Input: part model. Units: mm. Frame: model coordinates. A direction names the side the tool comes from. Round coordinates to 2 decimals unless told otherwise and drop trailing zeros. Loops run counter-clockwise (first coordinate to the right, second up) from the corner with the lowest first, then second, coordinate; pieces in that order, holes last. Notation, with made-up numbers: (-10.75, -16.75) -> (24.25, -16.75) arc R13 cw to (24.25, -2.75) -> close; hole circle Ø2 at (10.25, 12). An arc over 180 degrees is marked (long way). Answer in a Markdown table with one row per item. Add a question column.
Q1. Section A-A, the plane x = 0.9. Output: boundary loops of the cut face in (y, z), and give its area (3 significant figures).
Q2. Section D-D, the plane x = -0.65. Output: boundary loops of the cut face in (y, z).
Q3. Pin query (flat end, axial travel): pin 1 (0.8 mm diameter, centred on x = 0.5, y = -2, fed in from -Z); pin 2 (1.5 mm diameter, centred on y = -5, z = -3.5, fed in from -X). Return the tip coordinate at first contact, or that it passes through.
Q4. Section B-B, the plane z = -3.85. Output: boundary loops of the cut face in (x, y).
Q5. Ray query, L1, parallel to X at y = -5.75, z = -3.5; L2, parallel to Y at x = -0.15, z = -4.6; L3, parallel to Z at x = 1.05, y = -5. Return the intervals inside material, ascending. Write a range as from..to.
Q6. Section C-C, the plane y = -4.5. Output: boundary loops of the cut face in (x, z), and give its area (3 significant figures).
Q7. Reachability of faces 1 (the face through (0, -3, -2.346)), 2 (the face through (-0.362, -3, -3)), 3 (the face through (1.138, -3, -3)) from +Z, -Z, +X, -X, +Y, -Y: full face, straight path, thin tool, end or side. Return the list, or none.
```python
from build123d import *

# Parameters (mm, degrees)
F0_W     = 1.5
F0_H     = 2
F1_DEPTH = 6
F2_W     = 2.5
F2_H     = 3
F3_DEPTH = 1
F4_DEPTH = 1


with BuildPart() as f1:
    # F0 (on Front) → F1 (new body)
    with BuildSketch(Plane.XZ):
        with Locations((0.387931, -3.345636)):
            Rectangle(F0_W, F0_H)
    extrude(amount=F1_DEPTH)

    # F2 (on face) → F3 (join)
    with BuildSketch(Plane.XZ.offset(6)):
        with Locations((0.387931, -3.345636)):
            Rectangle(F2_W, F2_H)
    extrude(amount=F3_DEPTH)

    # F2 (on face) → F4 (join)
    with BuildSketch(Plane.XZ.offset(6)):
        with Locations((0.387931, -3.345636)):
            Rectangle(F2_W, F2_H)
    extrude(amount=F4_DEPTH)


solid = f1.part
```
Answer block:
| question | item | result |
|---|---|---|
| 1 | outline | (-7, -4.85) -> (-6, -4.85) -> (-6, -4.35) -> (0, -4.35) -> (0, -2.35) -> (-6, -2.35) -> (-6, -1.85) -> (-7, -1.85) -> close |
| 1 | area | 15.0 mm^2 |
| 2 | outline | (-7, -4.85) -> (-6, -4.85) -> (-6, -1.85) -> (-7, -1.85) -> close |
| 3 | pin 1 | z = -4.35 |
| 3 | pin 2 | x = -0.36 |
| 4 | outline | (-0.86, -7) -> (1.64, -7) -> (1.64, -6) -> (1.14, -6) -> (1.14, 0) -> (-0.36, 0) -> (-0.36, -6) -> (-0.86, -6) -> close |
| 5 | L1 | -0.36..1.14 |
| 5 | L2 | -7..-6 |
| 5 | L3 | -4.35..-2.35 |
| 6 | outline | (-0.36, -4.35) -> (1.14, -4.35) -> (1.14, -2.35) -> (-0.36, -2.35) -> close |
| 6 | area | 3.00 mm^2 |
| 7 | face 1 | +Z, +X, -X, +Y |
| 7 | face 2 | +Z, -Z, -X, +Y |
| 7 | face 3 | +Z, -Z, +X, +Y |
